from build123d import *

# Parameters (mm, degrees)
F0_R     = 1.5875
F1_DEPTH = 9.525
F2_SIZE  = 12.7
F3_R     = 3.175
F4_R     = 6.35


with BuildPart() as f1:
    # F0 (on Right) → F1 (new body, symmetric)
    with BuildSketch(Plane.YZ):
        with BuildLine():
            ThreePointArc((19.939, 0), (0, -19.939), (-19.939, 0))
            Line((-19.939, 0), (-24.7015, 0))
            Line((-24.7015, 0), (-31.0515, 0))
            Line((-31.0515, 0), (-31.0515, -4.7625))
            Line((-31.0515, -4.7625), (-24.7015, -4.7625))
            Line((-24.7015, -4.7625), (-24.7015, -24.7015))
            Line((-24.7015, -24.7015), (24.7015, -24.7015))
            Line((24.7015, -24.7015), (24.7015, -4.7625))
            ThreePointArc((24.7015, -4.7625), (28.0690960454, 3.3675960454), (19.939, 0))
        make_face()
        with Locations((24.7015, 0)):
            Circle(F0_R, mode=Mode.SUBTRACT)
    extrude(amount=F1_DEPTH, both=True)

    # F2
    f2_edges = [f1.edges().sort_by_distance(p)[0] for p in [
        (0, -24.7015, -24.7015),
        (0, 24.7015, -24.7015),
    ]]
    chamfer(f2_edges, length=F2_SIZE)

    # F3
    f3_edges = [f1.edges().sort_by_distance(p)[0] for p in [
        (0, 24.7015, -4.7625),
        (0, -24.7015, -4.7625),
    ]]
    fillet(f3_edges, radius=F3_R)

    # F4
    f4_edges = [f1.edges().sort_by_distance(p)[0] for p in [
        (0, 24.7015, -12.0015),
        (0, -24.7015, -12.0015),
    ]]
    fillet(f4_edges, radius=F4_R)


solid = f1.part
The listing builds one solid part. Answer for the finished solid, in the listing's coordinates (mm). A direction names the side the tool comes from. Coordinates: 2 decimals unless noted, no trailing zeros. Loops run counter-clockwise (first coordinate to the right, second up) from the corner with the lowest first, then second, coordinate; pieces in that order, holes last.
1) A tool of negligible diameter and unlimited length cuts with its end or side. For faces 4 (the face through (0, 24.702, -8)), 5 (the face through (0, -25, 0)), 6 (the face through (0, -24.702, -9)), 7 (the face through (-0.133, 26.216, 0.477)), from which of +Z, -Z, +X, -X, +Y, -Y can it reach the whole face along a straight path? Write none if from no direction.
2) Find section B-B on z = -3. Write down the section's boundary in (x, y) (1 decimal), then the cut area to 3 significant figures.
3) Find section C-C on y = 0. Write down the section's boundary in (x, z) (1 decimal).
4) Determine the mould class of faces 1 (the face through (0.133, -25.607, -5.717)), 2 (the face through (0.133, 0.438, -19.934)), 3 (the face through (-9.525, -3, -20)) for opening direction Y: pulls with the +Y half, pulls with the -Y half, needs draft (parallel to the pull), parting line crosses it, or undercut.
5) Find the intervals of material crossed by L1, parallel to Y at x = -7.5, z = -0.5; L2, parallel to Z at x = 2, y = 0.5; L3, parallel to Y at x = -4.75, z = -10, in increasing order.
6) Flat-ended cylindrical pins translate along their axes: pin 1 Ø1 at (x, z) = (6.5, 1) entering from +Y; pin 2 Ø2 at (x, y) = (5, 12) entering from +Z; pin 3 Ø5.5 at (x, y) = (-1.5, -26.5) entering from +Z. Find the tip coordinate at first contact, or state that the pin passes through.
Values:
1. face 4: -Z, +X, -X, +Y
1. face 5: +Z, +X, -X, -Y
1. face 6: -Z, +X, -X, -Y
1. face 7: +X, -X
2. outline: (-9.5, -31.1) - (9.5, -31.1) - (9.5, -19.7) - (-9.5, -19.7) - close; (-9.5, 19.7) - (9.5, 19.7) - (9.5, 28.4) - (-9.5, 28.4) - close
2. area: 382 mm2
3. outline: (-9.5, -24.7) - (9.5, -24.7) - (9.5, -19.9) - (-9.5, -19.9) - close
4. face 1: pulls with the -Y half
4. face 2: undercut
4. face 3: needs draft
5. L1: y = -31.05 to -19.93, 19.93 to 23.19, 26.21 to 29.44
5. L2: z = -24.7 to -19.93
5. L3: y = -24.67 to -17.25, 17.25 to 24.67
6. pin 1: stops at y = 29.44
6. pin 2: stops at z = -15.12
6. pin 3: stops at z = 0
